Input: dimensioned drawing with shaded views. Units: mm. Origin: part minimum x, y, z. A direction names the side the tool comes from. Give positions to 0.01 mm unless a question says otherwise; leave off trailing zeros. Loops run counter-clockwise (first coordinate to the right, second up) from the corner with the lowest first, then second, coordinate; pieces in that order, holes last. Notation, with made-up numbers: (-0.5, -25.5) -> (40.5, -25.5) arc R17 ccw to (40.5, -0.5) -> close; hole circle Ø6 at (44, -5.5). An arc over 180 degrees is marked (long way). One line per question, with ' | ' between items. Start each with the question number.
Item 1: Set-up query: the marked faces 1 and 2. Return all of +Z, -Z, +X, -X, +Y, -Y with unobstructed straight access to the full face (end or side cutting, diameter ignored); none if empty.
Item 2: Mould query, pull axis X, two halves, no side actions, for the marked faces 3, 4 and 5. Classes: released by +X, released by -X, zero draft, split by the parting line, or undercut.
Item 3: Section C-C on x = 37. Return loops of the section in (y, z), then the cut area to 3 significant figures.
Item 4: Section A-A on z = 18. Return loops of the section in (x, y), then the cut area to 3 significant figures.
Item 5: Pin query (flat end, axial travel): P1, Ø10, axis at x = 18, z = 15.5, coming from the +Y side; P2, Ø1.5, axis at x = 24, z = 21, coming from the -Y side; P3, Ø1, axis at x = 20.5, z = 15, coming from the +Y side. Return the tip coordinate at first contact, or that it passes through.
Item 6: Material intervals for line 1 along Y through (x, z) = (25, 12.5); line 2 along Z through (x, y) = (24.5, 23); line 3 along Y through (x, z) = (28.5, 19.25), sorted ascending. Write a range as [from, to].
Item 7: Section B-B on x = 9. Return loops of the section in (y, z), then the cut area to 3 significant figures.
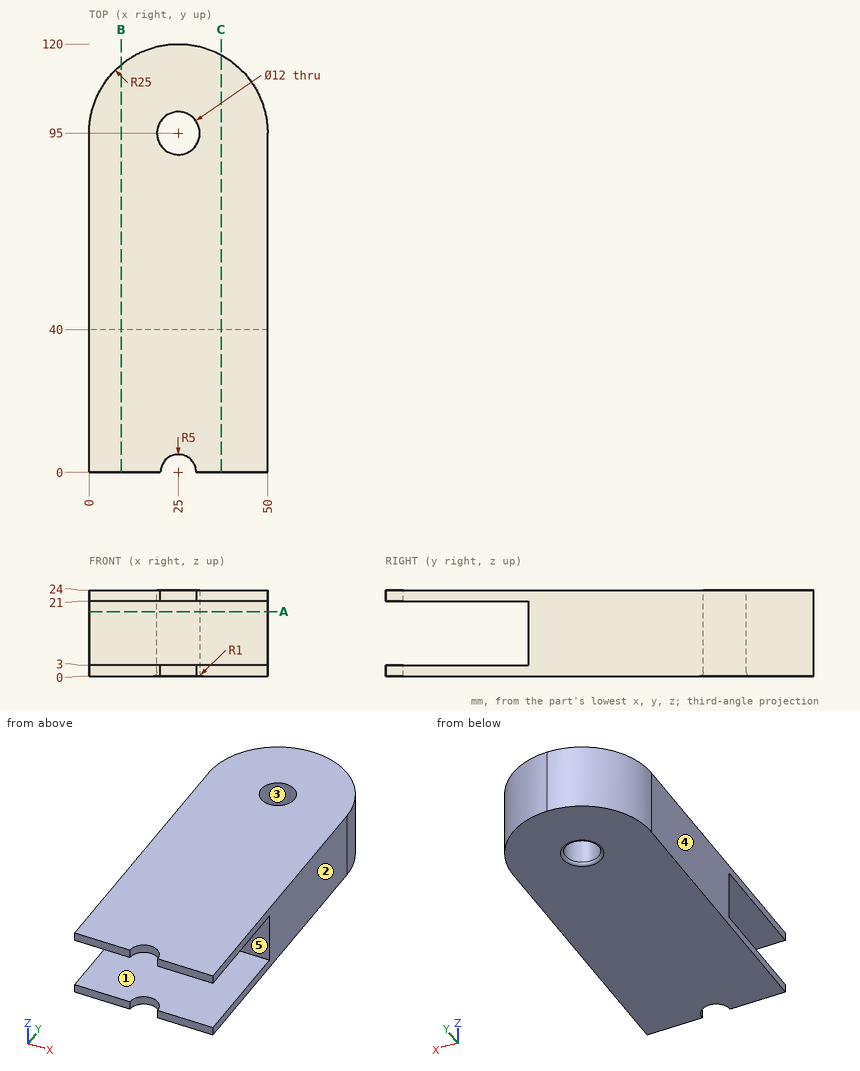
Result sheet:
1) face 1: +X, -X, -Y | face 2: +Z, -Z, +X, +Y, -Y
2) face 3: undercut | face 4: released by -X | face 5: zero draft
3) outline: (0, 0) -> (116.93, 0) -> (116.93, 24) -> (0, 24) -> (0, 21) -> (40, 21) -> (40, 3) -> (0, 3) -> close | area: 2,090 mm²
4) outline: (0, 40) -> (50, 40) -> (50, 95) arc R25 ccw to (0, 95) -> close; hole circle Ø12 at (25, 95) | area: 3,620 mm²
5) P1: stops at y = 119.92 | P2: stops at y = 4.68 | P3: stops at y = 119.68
6) line 1: y = [40, 89], [101, 120] | line 2: z = [0, 3], [21, 24] | line 3: y = [40, 90.13], [99.87, 119.75]
7) outline: (0, 0) -> (114.21, 0) -> (114.21, 24) -> (0, 24) -> (0, 21) -> (40, 21) -> (40, 3) -> (0, 3) -> close | area: 2,020 mm²
